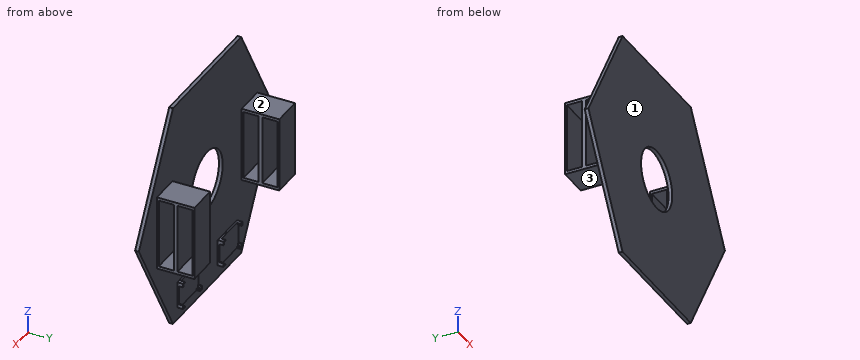
from build123d import *

# Parameters (mm, degrees)
BOSS_EXTRUDE1_DEPTH = 10
BOSS_EXTRUDE2_DEPTH = 15
SKETCH3_R           = 80
CUT_EXTRUDE1_DEPTH  = 10
SKETCH4_W           = 98
SKETCH4_H           = 71
BOSS_EXTRUDE3_DEPTH = 5
SKETCH5_W           = 80
SKETCH5_H           = 200
BOSS_EXTRUDE4_DEPTH = 100
SKETCH6_W           = 185
SKETCH6_H           = 40
CUT_EXTRUDE2_DEPTH  = 80


with BuildPart() as part:
    # Sketch1 → Boss-Extrude1 (new body)
    with BuildSketch(Plane(origin=(0, 0, 0), x_dir=(1, 0, 0), z_dir=(0, 1, 0))):
        Polygon((350, 0), (175, 303.108891325), (-175, 303.108891325), (-350, 0), (-175, -303.108891325), (175, -303.108891325), align=None)
    extrude(amount=BOSS_EXTRUDE1_DEPTH)

    # Sketch2 → Boss-Extrude2 (add)
    with BuildSketch(Plane(origin=(0, 10, 0), x_dir=(1, 0, 0), z_dir=(0, 1, 0))):
        Polygon((54.532889038, 198.679724117), (64.532889038, 198.679724117), (64.532889038, 201.679724117), (57.532889038, 201.679724117), (57.532889038, 208.679724117), (54.532889038, 208.679724117), align=None)
        Polygon((142.532889038, 201.679724117), (142.532889038, 198.679724117), (152.532889038, 198.679724117), (152.532889038, 208.679724117), (149.532889038, 208.679724117), (149.532889038, 201.679724117), align=None)
        Polygon((54.532889038, 259.679724117), (57.532889038, 259.679724117), (57.532889038, 266.679724117), (64.532889038, 266.679724117), (64.532889038, 269.679724117), (54.532889038, 269.679724117), align=None)
        Polygon((149.532889038, 259.679724117), (152.532889038, 259.679724117), (152.532889038, 269.679724117), (142.532889038, 269.679724117), (142.532889038, 266.679724117), (149.532889038, 266.679724117), align=None)
        Polygon((-64.532889038, 201.679724117), (-64.532889038, 198.679724117), (-54.532889038, 198.679724117), (-54.532889038, 208.679724117), (-57.532889038, 208.679724117), (-57.532889038, 201.679724117), align=None)
        Polygon((-142.532889038, 198.679724117), (-142.532889038, 201.679724117), (-149.532889038, 201.679724117), (-149.532889038, 208.679724117), (-152.532889038, 208.679724117), (-152.532889038, 198.679724117), align=None)
        Polygon((-152.532889038, 259.679724117), (-149.532889038, 259.679724117), (-149.532889038, 266.679724117), (-142.532889038, 266.679724117), (-142.532889038, 269.679724117), (-152.532889038, 269.679724117), align=None)
        Polygon((-57.532889038, 259.679724117), (-54.532889038, 259.679724117), (-54.532889038, 269.679724117), (-64.532889038, 269.679724117), (-64.532889038, 266.679724117), (-57.532889038, 266.679724117), align=None)
    extrude(amount=BOSS_EXTRUDE2_DEPTH)

    # Sketch3 → Cut-Extrude1 (cut)
    with BuildSketch(Plane(origin=(0, 10, 0), x_dir=(1, 0, 0), z_dir=(0, 1, 0))):
        with Locations(Location((0, 0, 0), (0, 0, 270))):
            Circle(SKETCH3_R)
    extrude(amount=-CUT_EXTRUDE1_DEPTH, mode=Mode.SUBTRACT)

    # Sketch4 → Boss-Extrude3 (add)
    with BuildSketch(Plane(origin=(0, 10, 0), x_dir=(1, 0, 0), z_dir=(0, 1, 0))):
        with Locations((-103.532889038, 234.179724117)):
            Rectangle(SKETCH4_W, SKETCH4_H)
        with Locations((103.532889038, 234.179724117)):
            Rectangle(SKETCH4_W, SKETCH4_H)
    extrude(amount=BOSS_EXTRUDE3_DEPTH)

    # Sketch5 → Boss-Extrude4 (add)
    with BuildSketch(Plane(origin=(0, 10, 0), x_dir=(1, 0, 0), z_dir=(0, 1, 0))):
        with Locations((-217.647690378, 0)):
            Rectangle(SKETCH5_W, SKETCH5_H)
    boss_extrude4 = extrude(amount=BOSS_EXTRUDE4_DEPTH)

    # Sketch6 → Cut-Extrude2 (cut)
    with BuildSketch(Plane.ZY.offset(257.647690378)):
        with Locations((0, 35)):
            Rectangle(SKETCH6_W, SKETCH6_H)
        with Locations((0, 85)):
            Rectangle(SKETCH6_W, SKETCH6_H)
    cut_extrude2 = extrude(amount=-CUT_EXTRUDE2_DEPTH, mode=Mode.SUBTRACT)

    # Mirror1: Boss-Extrude4, Cut-Extrude2 across plane
    add(boss_extrude4.mirror(Plane(origin=(0, 0, 0), x_dir=(0, 0, 1), z_dir=(1, 0, 0))))
    add(cut_extrude2.mirror(Plane(origin=(0, 0, 0), x_dir=(0, 0, 1), z_dir=(1, 0, 0))), mode=Mode.SUBTRACT)


solid = part.part
For this review, take the finished solid that the model builds, in its own axes (mm). Face numbers are marked on the shaded views. A direction names the side the tool comes from. Coordinates: 2 decimals unless noted, no trailing zeros. Order: outer loops, then holes, each group sorted by start corner. A loop starts at its lowest first (then second) coordinate and runs counter-clockwise, first axis right, second up. Notation, with made-up numbers: (-31, 35) -> (10, 35) arc R25 cw to (10, 57) -> close; hole circle Ø10 at (-18, -26.5). An arc over 180 degrees is marked (long way). Return JSON: item names as keys, results as strings.
1. We need section A-A on x = 0. Write out the cut boundary in (y, z).
Answer block:
{"outline": "(0, -303.11) -> (10, -303.11) -> (10, -80) -> (0, -80) -> close; (0, 80) -> (10, 80) -> (10, 303.11) -> (0, 303.11) -> close"}
2. We need section B-B on y = 77. Write out the cut boundary in (x, z).
Answer block:
{"outline": "(-257.65, -100) -> (-177.65, -100) -> (-177.65, -92.5) -> (-257.65, -92.5) -> close; (-257.65, 92.5) -> (-177.65, 92.5) -> (-177.65, 100) -> (-257.65, 100) -> close; (177.65, -100) -> (257.65, -100) -> (257.65, -92.5) -> (177.65, -92.5) -> close; (177.65, 92.5) -> (257.65, 92.5) -> (257.65, 100) -> (177.65, 100) -> close"}
3. Machinability: for the marked faces 1, 2 and 3, which of the approach directions +Z, -Z, +X, -X, +Y, -Y give a long, thin tool a straight path to every point of the face, cutting with its end or side? Answer none if there is none.
Answer block:
{"face 1": "+Z, -Z, +X, -X, -Y", "face 2": "+Z, +X, -X, +Y", "face 3": "-Z, +X, -X, +Y"}
4. For line 1 (Y direction, x = -198.5, z = 67.5); line 2 (X direction, y = 5.75, z = 0); line 3 (X direction, y = 60, z = 52), list the stretches that pass through material, from the lowest coordinate up. Write a range as from..to.
Answer block:
{"line 1": "0..15, 55..65, 105..110", "line 2": "-350..-80, 80..350", "line 3": "-257.65..-177.65, 177.65..257.65"}
5. We need section D-D on x = 135. Write out the cut boundary in (y, z), and give its area (3 significant figures).
Answer block:
{"outline": "(0, -303.11) -> (10, -303.11) -> (10, -269.68) -> (15, -269.68) -> (15, -198.68) -> (10, -198.68) -> (10, 303.11) -> (0, 303.11) -> close", "area": "6,420 mm²"}
6. For pin 1 Ø2 at (x, y) = (60, 22.5) entering from -Z; pin 2 Ø7.5 at (y, z) = (19, -206.5) entering from -X; pin 3 Ø24 at (x, y) = (-223, 36.5) entering from -Z; pin 4 Ø12 at (x, z) = (194, 110) entering from -Y, all flat-tipped, find the tip position at first contact; note any pin that passes through.
Answer block:
{"pin 1": "z = -269.68", "pin 2": "x = -152.53", "pin 3": "z = -100", "pin 4": "y = 0"}
7. We need section C-C on z = -72.5. State how many separate pieces and enclosed holes the cut face has, and give its area (3 significant figures).
Answer block:
{"separate pieces": "6", "enclosed holes": "0", "area": "8,690 mm²"}
